from build123d import *

# Parameters (mm, degrees)
SKETCH1_W           = 152.4
SKETCH1_H           = 76.2
BOSS_EXTRUDE1_DEPTH = 76.2
SKETCH2_W           = 2.54
SKETCH2_H           = 10.16
SKETCH5_W           = 19.05
SKETCH5_H           = 19.05
BOSS_EXTRUDE2_DEPTH = 0.254


with BuildPart() as part:
    # Sketch1 → Boss-Extrude1 (new body)
    with BuildSketch(Plane(origin=(0, 0, 0), x_dir=(1, 0, 0), z_dir=(0, 1, 0))):
        Rectangle(SKETCH1_W, SKETCH1_H)
    extrude(amount=BOSS_EXTRUDE1_DEPTH)

    # Sweep1: sweep along a path in Sketch4
    with BuildLine(Plane.XY) as sweep1_path:
        Line((-62.23, 76.2), (-62.23, 78.74))
        ThreePointArc((-62.23, 78.74), (-61.932876443, 79.556340264), (-61.180533186, 79.990705846))
        Line((-61.180533186, 79.990705846), (-48.673474722, 82.196037703))
    # Sketch2 → Sweep1 (sweep)
    with BuildSketch(Plane(origin=(0, 76.2, 0), x_dir=(1, 0, 0), z_dir=(0, 1, 0))):
        with Locations((-62.23, 20.32)):
            Rectangle(SKETCH2_W, SKETCH2_H)
        with Locations((-62.23, -20.32)):
            Rectangle(SKETCH2_W, SKETCH2_H)
    sweep(path=sweep1_path.line)

    # Sketch5 → Boss-Extrude2 (add)
    with BuildSketch(Plane(origin=(0, 76.2, 0), x_dir=(1, 0, 0), z_dir=(0, 1, 0))):
        with Locations((-59.055, 20.6375)):
            Rectangle(SKETCH5_W, SKETCH5_H)
    extrude(amount=BOSS_EXTRUDE2_DEPTH)


solid = part.part
Geometry: final body of the model. Coordinates: model frame, mm. A direction names the side the tool comes from. Give positions to 0.01 mm unless a question says otherwise; leave off trailing zeros. Write each loop counter-clockwise with the first axis right and the second up, starting at its lowest first coordinate (ties: lowest second). Pieces come first, ordered by that corner, then holes. Notation, with made-up numbers: (19.25, 50) - (36.25, 50) arc R38 ccw to (36.25, 89) - close; hole circle Ø1 at (56.25, 17.25). An arc over 180 degrees is marked (long way). Return JSON: item names as keys, results as strings. Group by question number.
1) Section D-D on z = -27. Return the cut outline in (x, y).
2) First-contact query: P1, Ø5, axis at x = 21, z = -24.5, coming from the +Y side; P2, Ø7.5, axis at x = -54.5, y = 81, coming from the +Z side; P3, Ø2, axis at x = -59, y = 78.5, coming from the -Z side. Flat tips, straight axial feed; report the tip coordinate or a pass-through.
3) Set-up query: faces 1 (the flat face through (-58, 80, 25.4)), 2 (the flat face through (-54.619, 79.858, -20.249)), 3 (the flat face through (76.2, 38, 1)), 4 (the flat face through (-56, 81, 15.24)), 5 (the flat face through (-56, 81, -25.4)). Return all of +Z, -Z, +X, -X, +Y, -Y with unobstructed straight access to the full face (end or side cutting, diameter ignored); none if empty.
4) Mould query, pull axis Y, two halves, no side actions, for faces 6 (the flat face through (-58, 80, -15.24)), 7 (the flat face through (-1, 0, -1)), 8 (the flat face through (-55.06, 82.36, -20.39)), 9 (the flat face through (-54.619, 79.858, 20.391)). Classes: released by +Y, released by -Y, zero draft, split by the parting line, or undercut.
5) Line query: line 1 (Y direction, x = 22.5, z = -31.5); line 2 (X direction, y = 76.5, z = 18.5). Output: solid intervals per line, ascending.
6) Section C-C on x = -32. Return the cut outline in (y, z), plus the area to 3 significant figures.
7) Section B-B on x = -55. Return the cut outline in (y, z).
8) Section A-A on z = 17.5. Return the cut outline in (x, y).
Filled in:
{
 "1": {"outline": "(-76.2, 0) - (76.2, 0) - (76.2, 76.2) - (-49.53, 76.2) - (-49.53, 76.45) - (-68.58, 76.45) - (-68.58, 76.2) - (-76.2, 76.2) - close"},
 "2": {"P1": "stops at y = 76.2", "P2": "stops at z = 25.4", "P3": "stops at z = -25.4"},
 "3": {"face 1": "+Z, +X, -X, +Y", "face 2": "+Z, -Z, +X", "face 3": "+Z, -Z, +X, +Y, -Y", "face 4": "+X, -X, +Y", "face 5": "-Z, +X, -X, +Y"},
 "4": {"face 6": "zero draft", "face 7": "released by -Y", "face 8": "released by +Y", "face 9": "undercut"},
 "5": {"line 1": "y = 0 to 76.2", "line 2": "x = -63.5 to -60.96"},
 "6": {"outline": "(0, -38.1) - (76.2, -38.1) - (76.2, 38.1) - (0, 38.1) - close", "area": "5,810 mm^2"},
 "7": {"outline": "(0, -38.1) - (76.2, -38.1) - (76.2, -30.16) - (76.45, -30.16) - (76.45, -11.11) - (76.2, -11.11) - (76.2, 38.1) - (0, 38.1) - close; (79.79, -25.4) - (82.37, -25.4) - (82.37, -15.24) - (79.79, -15.24) - close; (79.79, 15.24) - (82.37, 15.24) - (82.37, 25.4) - (79.79, 25.4) - close"},
 "8": {"outline": "(-76.2, 0) - (76.2, 0) - (76.2, 76.2) - (-60.96, 76.2) - (-60.96, 78.74) - (-48.45, 80.95) - (-48.89, 83.45) - (-61.4, 81.24) arc R2.54 ccw to (-63.5, 78.74) - (-63.5, 76.2) - (-76.2, 76.2) - close"}
}
